Verification items for the finished model (mm, model axes). A direction names the side the tool comes from. Give positions to 0.01 mm unless a question says otherwise; leave off trailing zeros. Write each loop counter-clockwise with the first axis right and the second up, starting at its lowest first coordinate (ties: lowest second). Pieces come first, ordered by that corner, then holes. Notation, with made-up numbers: (27.5, 37.25) -> (66.5, 37.25) arc R30 cw to (66.5, 71.25) -> close; hole circle Ø1 at (38.25, 58). An arc over 180 degrees is marked (long way). Answer as CSV lines item,"result".
```python
from build123d import *

# Parameters (mm, degrees)
F1_DEPTH = 15
F2_R     = 2.5
F3_DEPTH = 7.001
F4_SIZE  = 2


with BuildPart() as f1:
    # F0 (on Top) → F1 (new body)
    with BuildSketch(Plane.XY):
        with BuildLine():
            Line((-47.371286, 2), (-47.371286, 0))
            Line((-47.371286, 0), (-34.371286, 0))
            ThreePointArc((-34.371286, 0), (-29.382447, 4.999988), (-24.371336, 0.022323))
            Line((-24.371336, 0.022323), (-11.371336, 0.022323))
            Line((-11.371336, 0.022323), (-11.371336, 2.022323))
            Line((-11.371336, 2.022323), (-22.669778, 2.022323))
            ThreePointArc((-22.669778, 2.022323), (-29.382938, 6.99999), (-36.07949, 2))
            Line((-36.07949, 2), (-47.371286, 2))
        make_face()
    extrude(amount=F1_DEPTH)

    # F2 (on Front) → F3 (cut, through all)
    with BuildSketch(Plane.XZ):
        with Locations((-41.871286, 7.5)):
            Circle(F2_R)
        with Locations((-16.871336, 7.5)):
            Circle(F2_R)
    extrude(amount=-F3_DEPTH, mode=Mode.SUBTRACT)

    # F4
    f4_edges = [f1.edges().sort_by_distance(p)[0] for p in [
        (-11.371336, 1.022323, 15),
        (-47.371286, 1, 15),
        (-11.371336, 1.022323, 0),
        (-47.371286, 1, 0),
    ]]
    chamfer(f4_edges, length=F4_SIZE)


solid = f1.part
```
1) Scan lines: line 1 along Y through (x, z) = (-44, 11); line 2 along X through (y, z) = (0.75, 11); line 3 along X through (y, z) = (2.5, 13.25). Record each from-to range of solid material in increasing order.
Reported:
line 1,"0 to 2"
line 2,"-47.37 to -34.31, -24.43 to -11.37"
line 3,"-35.91 to -33.7, -25.04 to -22.83"
2) Tool access check on faces 1 (the cylindrical face through (-29.3, 7, 7.4)), 2 (the flat face through (-39, 2, 7)), 3 (the flat face through (-19.5, 2.022, 9.1)). Record the directions out of +Z, -Z, +X, -X, +Y, -Y that give a thin tool (end or side, any length) a straight path to the whole face; none if there is none.
Reported:
face 1,"+Z, -Z, +Y"
face 2,"+Z, -Z, -X, +Y"
face 3,"+Z, -Z, +X, +Y"
3) Depth check by flat-ended pin: pin 1 (1.5 mm diameter, centred on x = -42, y = 4, fed in from +Z); pin 2 (9 mm diameter, centred on x = -15, z = 7, fed in from +Y); pin 3 (4 mm diameter, centred on x = -17, z = 10.5, fed in from -Y); pin 4 (1.5 mm diameter, centred on y = 4, z = 6, fed in from +X). Enter the tip coordinate at first touch or a pass-through.
Reported:
pin 1,"through"
pin 2,"y = 2.02"
pin 3,"y = 0.02"
pin 4,"x = -23.17"
4) Section check D-D (y = 2.75). Record the boundary of the cut face in (x, z).
Reported:
outline,"(-35.81, 0) -> (-33.55, 0) -> (-33.55, 15) -> (-35.81, 15) -> close; (-25.2, 0) -> (-22.93, 0) -> (-22.93, 15) -> (-25.2, 15) -> close"
5) Draft check along X on faces 4 (the flat face through (-46.36, 1.01, 14.01)), 5 (the flat face through (-11.371, 1, 7)), 6 (the cylindrical face through (-14.562, 1.008, 6.542)), 7 (the cylindrical face through (-29.5, 5, 7.4)). Enter one of: +X half, -X half, draft (parallel to the pull), parting line (faces both ways), or undercut.
Reported:
face 4,"-X half"
face 5,"+X half"
face 6,"undercut"
face 7,"undercut"
6) Section check A-A (z = 7.5). Record the boundary of the cut face in (x, y), and give its area (3 significant figures).
Reported:
outline,"(-47.37, 0) -> (-44.37, 0) -> (-44.37, 2) -> (-47.37, 2) -> close; (-39.37, 0) -> (-34.37, 0) arc R5 cw to (-24.37, 0.02) -> (-19.37, 0.02) -> (-19.37, 2.02) -> (-22.67, 2.02) arc R7 ccw to (-36.08, 2) -> (-39.37, 2) -> close; (-14.37, 0.02) -> (-11.37, 0.02) -> (-11.37, 2.02) -> (-14.37, 2.02) -> close"
area,"62.0 mm²"
7) Section check C-C (z = 10.5). Record the boundary of the cut face in (x, y).
Reported:
outline,"(-47.37, 0) -> (-34.37, 0) arc R5 cw to (-24.37, 0.02) -> (-11.37, 0.02) -> (-11.37, 2.02) -> (-22.67, 2.02) arc R7 ccw to (-36.08, 2) -> (-47.37, 2) -> close"
8) Section check B-B (x = -17.5). Record the boundary of the cut face in (y, z), and give its area (3 significant figures).
Reported:
outline,"(0.02, 0) -> (2.02, 0) -> (2.02, 5.08) -> (0.02, 5.08) -> close; (0.02, 9.92) -> (2.02, 9.92) -> (2.02, 15) -> (0.02, 15) -> close"
area,"20.3 mm²"
